Can you work these out from the model? Positions are in its coordinate system, mm. A direction names the side the tool comes from. Give positions to 0.01 mm unless a question says otherwise; leave off trailing zeros. Loops run counter-clockwise (first coordinate to the right, second up) from the corner with the lowest first, then second, coordinate; pieces in that order, holes last. Notation, with made-up numbers: (48.5, 60.5) -> (93.5, 60.5) arc R11 cw to (93.5, 66.5) -> close; hole circle Ø6 at (23, 1.25). An arc over 180 degrees is marked (long way). Use CSV: the item, a comma, the result in double quotes.
Autodesk Inventor part; units mm, degrees
ref_plane "YZ Plane" through (0, 0, 0) normal (1, 0, 0) x (0, 1, 0)
ref_plane "XZ Plane" through (0, 0, 0) normal (0, 1, 0) x (-1, 0, 0)
ref_plane "XY Plane" through (0, 0, 0) normal (0, 0, 1) x (1, 0, 0)
sketch "Sketch1" plane through (0, 0, 0) normal (0, 0, 1) x (1, 0, 0)
  line L0 (0, 53.34) -> (96.52, 53.34)
  line L1 (96.52, 53.34) -> (99.06, 50.8)
  line L2 (99.06, 50.8) -> (99.06, 40.64)
  line L3 (99.06, 40.64) -> (101.6, 38.1)
  line L4 (101.6, 38.1) -> (101.6, 3.81)
  line L5 (99.06, 0) -> (0, 0)
  line L6 (0, 0) -> (0, 53.34)
  line L7 (101.6, 3.81) -> (99.06, 1.27)
  line L8 (99.06, 1.27) -> (99.06, 0)
  line L9 (96.9093, 54.2798) -> (-0.9398, 54.2798)
  line L10 (-0.9398, 54.2798) -> (-0.9398, -0.9398)
  line L11 (-0.9398, -0.9398) -> (99.9998, -0.9398)
  line L12 (99.9998, -0.9398) -> (99.9998, 0.8807)
  line L13 (99.9998, 0.8807) -> (102.5398, 3.4207)
  line L14 (102.5398, 3.4207) -> (102.5398, 38.4893)
  line L15 (102.5398, 38.4893) -> (99.9998, 41.0293)
  line L16 (99.9998, 41.0293) -> (99.9998, 51.1893)
  line L17 (99.9998, 51.1893) -> (96.9093, 54.2798)
  line L18 (96.6042, 53.5432) -> (-0.2032, 53.5432)
  line L19 (-0.2032, 53.5432) -> (-0.2032, -0.2032)
  line L20 (-0.2032, -0.2032) -> (99.2632, -0.2032)
  line L21 (99.2632, -0.2032) -> (99.2632, 1.1858)
  line L22 (99.2632, 1.1858) -> (101.8032, 3.7258)
  line L23 (101.8032, 3.7258) -> (101.8032, 38.1842)
  line L24 (101.8032, 38.1842) -> (99.2632, 40.7242)
  line L25 (99.2632, 40.7242) -> (99.2632, 50.8842)
  line L26 (99.2632, 50.8842) -> (96.6042, 53.5432)
  point P0 (0, 0)
  dimension "d0" = 96.52
  dimension "d1" = 53.34
  dimension "d4" = 99.06
  dimension "d5" = 50.8
  dimension "d6" = 101.6
  dimension "d7" = 40.64
  dimension "d8" = 38.1
  dimension "d9" = 99.06
  dimension "d10" = 1.27
  dimension "d11" = 3.81
  dimension "d15" = 0.2032
  dimension "d18" = 0.7366
extrude "Extrusion2" add sketch "Sketch1" along normal blind 2.54 contours L17 L16 L15 L14 L13 L12 L11 L10 L9
sketch "Sketch2" plane through (0, 0, 0) normal (0, 0, 1) x (1, 0, 0)
  line L0 (0, 53.34) -> (96.52, 53.34)
  line L1 (96.52, 53.34) -> (99.06, 50.8)
  line L2 (99.06, 50.8) -> (99.06, 40.64)
  line L3 (99.06, 40.64) -> (101.6, 38.1)
  line L4 (101.6, 38.1) -> (101.6, 3.81)
  line L5 (99.06, 0) -> (0, 0)
  line L6 (0, 0) -> (0, 53.34)
  line L7 (101.6, 3.81) -> (99.06, 1.27)
  line L8 (99.06, 1.27) -> (99.06, 0)
  line L9 (96.9093, 54.2798) -> (-0.9398, 54.2798)
  line L10 (-0.9398, 54.2798) -> (-0.9398, -0.9398)
  line L11 (-0.9398, -0.9398) -> (99.9998, -0.9398)
  line L12 (99.9998, -0.9398) -> (99.9998, 0.8807)
  line L13 (99.9998, 0.8807) -> (102.5398, 3.4207)
  line L14 (102.5398, 3.4207) -> (102.5398, 38.4893)
  line L15 (102.5398, 38.4893) -> (99.9998, 41.0293)
  line L16 (99.9998, 41.0293) -> (99.9998, 51.1893)
  line L17 (99.9998, 51.1893) -> (96.9093, 54.2798)
  line L18 (96.6042, 53.5432) -> (-0.2032, 53.5432)
  line L19 (-0.2032, 53.5432) -> (-0.2032, -0.2032)
  line L20 (-0.2032, -0.2032) -> (99.2632, -0.2032)
  line L21 (99.2632, -0.2032) -> (99.2632, 1.1858)
  line L22 (99.2632, 1.1858) -> (101.8032, 3.7258)
  line L23 (101.8032, 3.7258) -> (101.8032, 38.1842)
  line L24 (101.8032, 38.1842) -> (99.2632, 40.7242)
  line L25 (99.2632, 40.7242) -> (99.2632, 50.8842)
  line L26 (99.2632, 50.8842) -> (96.6042, 53.5432)
  line L27 (4.1402, 4.1402) -> (4.1402, 49.1998)
  circle A0 centre (15.24, 50.8) radius 1.5875
  circle A1 centre (13.97, 2.54) radius 1.5875
  line L28 (13.7585, 47.9425) -> (16.8275, 47.9425)
  line L29 (16.8275, 47.9425) -> (18.0848, 49.1998)
  line L30 (13.7585, 47.9425) -> (12.5012, 49.1998)
  line L31 (4.1402, 49.1998) -> (12.5012, 49.1998)
  line L32 (18.0848, 49.1998) -> (87.3252, 49.1998)
  line L33 (12.3825, 5.3344) -> (15.5575, 5.3344)
  line L34 (15.5575, 5.3344) -> (16.7517, 4.1402)
  line L35 (12.3825, 5.3344) -> (11.1883, 4.1402)
  line L36 (91.8972, 4.1402) -> (16.7517, 4.1402)
  line L37 (11.1883, 4.1402) -> (4.1402, 4.1402)
  line L38 (91.8972, 46.2153) -> (91.8972, 4.1402)
  circle A2 centre (90.17, 50.8) radius 1.5875
  circle A3 centre (96.52, 2.54) radius 1.5875
  line L39 (90.17, 47.9425) -> (88.5825, 47.9425)
  line L40 (88.5825, 47.9425) -> (87.3252, 49.1998)
  line L41 (90.17, 47.9425) -> (91.8972, 46.2153)
  point P0 (0, 0)
  point P1 (0, 1.4137)
  dimension "d19" = 96.52
  dimension "d20" = 53.34
  dimension "d21" = 99.06
  dimension "d22" = 50.8
  dimension "d23" = 101.6
  dimension "d24" = 40.64
  dimension "d25" = 38.1
  dimension "d26" = 99.06
  dimension "d27" = 1.27
  dimension "d28" = 3.81
  dimension "d29" = 0.2032
  dimension "d30" = 0.7366
  dimension "d70" = 13.97
  dimension "d71" = 2.54
  dimension "d72" = 3.175
  dimension "d73" = 50.8
  dimension "d74" = 3.175
  dimension "d75" = 15.24
  dimension "d135" = 2.54
  dimension "d136" = 1.27
  dimension "d146" = 4.1402
  dimension "d148" = 91.8972
  dimension "d150" = 3.175
  dimension "d151" = 3.175
  dimension "d152" = 90.17
  dimension "d153" = 50.8
  dimension "d154" = 1.27
  dimension "d155" = 2.54
  dimension "d156" = 96.52
extrude "Extrusion3" add sketch "Sketch2" against normal blind 2.54 contours L0 L1 L2 L3 L4 L7 L8 L5 L6 | L17 L16 L15 L14 L13 L12 L11 L10 L9 | L26 L25 L24 L23 L22 L21 L20 L19 L18
sketch "Sketch4" plane through (0, 0, 2.54) normal (0, 0, 1) x (1, 0, 0)
  line L0 (-0.2032, -0.2032) -> (-0.2032, 53.5432)
  line L1 (-0.9398, -0.9398) -> (-0.9398, 54.2798)
  line L2 (-0.2032, 12.446) -> (-0.9398, 12.446)
  line L3 (-0.2032, 2.8575) -> (-0.9398, 2.8575)
  line L4 (-0.2032, 32.004) -> (-0.9398, 32.004)
  line L5 (-0.2032, 44.196) -> (-0.9398, 44.196)
  point P0 (0, 0)
  dimension "d35" = 12.446
  dimension "d36" = 2.8575
  dimension "d37" = 32.004
  dimension "d38" = 44.196
extrude "Extrusion4" cut sketch "Sketch4" against normal blind 2.286 contours L3 L1 L2 L0 | L4 L1 L5 L0
sketch "Sketch5" plane through (0, 0, 0) normal (0, 0, 1) x (1, 0, 0)
  line L0 (25.4, 3.3338) -> (92.71, 3.3338)
  line L1 (92.71, 3.3338) -> (92.71, 1.7463)
  line L2 (92.71, 1.7463) -> (25.4, 1.7463)
  line L3 (25.4, 1.7463) -> (25.4, 3.3338)
  line L4 (17.78, 51.5938) -> (87.63, 51.5938)
  line L5 (87.63, 51.5938) -> (87.63, 50.0063)
  line L6 (87.63, 50.0063) -> (17.78, 50.0062)
  line L7 (17.78, 50.0062) -> (17.78, 51.5938)
  line L8 (-0.2032, 53.5432) -> (-0.2032, -0.2032)
  line L9 (-0.2032, 12.065) -> (11.2268, 12.065)
  line L10 (11.2268, 12.065) -> (11.2268, 1.6002)
  line L11 (11.2268, 1.6002) -> (-0.2032, 1.6002)
  line L12 (-0.2032, 1.6002) -> (-0.2032, 12.065)
  line L13 (1.6002, 12.065) -> (1.6002, 1.6002)
  line L14 (4.1402, 4.1402) -> (4.1402, 49.1998)
  line L15 (4.1402, 49.1998) -> (12.5012, 49.1998)
  line L16 (91.8972, 4.1402) -> (16.7517, 4.1402)
  line L17 (99.2632, 50.8842) -> (96.6042, 53.5432)
  line L18 (96.6042, 53.5432) -> (-0.2032, 53.5432)
  line L19 (-0.2032, 53.5432) -> (-0.2032, -0.2032)
  line L20 (-0.2032, -0.2032) -> (99.2632, -0.2032)
  line L21 (99.2632, -0.2032) -> (99.2632, 1.1858)
  line L22 (99.2632, 1.1858) -> (101.8032, 3.7258)
  line L23 (101.8032, 3.7258) -> (101.8032, 38.1842)
  line L24 (101.8032, 38.1842) -> (99.2632, 40.7242)
  line L25 (99.2632, 40.7242) -> (99.2632, 50.8842)
  line L26 (91.8972, 4.1402) -> (16.7517, 4.1402)
  line L27 (4.1402, 4.1402) -> (4.1402, 49.1998)
  line L28 (1.6002, 44.4853) -> (4.1402, 47.0253)
  line L29 (99.2632, 40.7242) -> (99.2632, 50.8842)
  line L30 (1.6002, 31.7147) -> (4.1402, 29.1747)
  line L31 (1.6002, 31.7147) -> (1.6002, 44.4853)
  line L32 (4.1402, 47.0253) -> (4.1402, 29.1747)
  line L33 (12.5012, 49.1998) -> (13.7585, 47.9425)
  line L34 (13.7585, 47.9425) -> (16.8275, 47.9425)
  line L35 (16.8275, 47.9425) -> (18.0848, 49.1998)
  line L36 (18.0848, 49.1998) -> (87.3252, 49.1998)
  line L37 (11.1883, 4.1402) -> (4.1402, 4.1402)
  line L38 (16.7517, 4.1402) -> (15.5575, 5.3344)
  line L39 (15.5575, 5.3344) -> (12.3825, 5.3344)
  line L40 (12.3825, 5.3344) -> (11.1883, 4.1402)
  line L41 (15.5575, 5.3344) -> (12.3825, 5.3344)
  line L42 (97.79, 51.5938) -> (92.71, 51.5938)
  line L43 (92.71, 51.5938) -> (92.71, 6.35)
  line L44 (92.71, 6.35) -> (97.79, 6.35)
  line L45 (97.79, 6.35) -> (97.79, 51.5938)
  line L46 (91.8972, 46.2153) -> (91.8972, 4.1402)
  line L47 (87.3252, 49.1998) -> (88.5825, 47.9425)
  line L48 (88.5825, 47.9425) -> (90.17, 47.9425)
  line L49 (90.17, 47.9425) -> (91.8972, 46.2153)
  point P0 (0, 0)
  point P1 (61.8998, 4.1402)
  dimension "d41" = 1.5875
  dimension "d42" = 25.4
  dimension "d43" = 92.71
  dimension "d44" = 17.78
  dimension "d45" = 87.63
  dimension "d46" = 1.5875
  dimension "d47" = 51.5938
  dimension "d48" = 1.7463
  dimension "d51" = 0
  dimension "d52" = 12.065
  dimension "d54" = 11.43
  dimension "d97" = 2.54
  dimension "d101" = 2.54
  dimension "d102" = 2.54
  dimension "d142" = 5.08
  dimension "d143" = 0
  dimension "d145" = 6.35
  dimension "d149" = 92.71
extrude "Extrusion5" cut sketch "Sketch5" against normal blind 2.159 contours L0 L1 L2 L3 | L4 L5 L6 L7 | L45 L44 L43 L42
sketch "Sketch7" plane through (0, 0, 0) normal (0, 0, 1) x (1, 0, 0)
  line L0 (25.4, 3.3338) -> (64.77, 3.3338)
  line L1 (64.77, 3.3338) -> (64.77, 1.7463)
  line L2 (64.77, 1.7463) -> (25.4, 1.7463)
  line L3 (25.4, 1.7463) -> (25.4, 3.3338)
  line L4 (17.78, 51.5938) -> (64.77, 51.5938)
  line L5 (64.77, 51.5938) -> (64.77, 50.0062)
  line L6 (64.77, 50.0062) -> (17.78, 50.0062)
  line L7 (17.78, 50.0062) -> (17.78, 51.5938)
  line L8 (-0.2032, 53.5432) -> (-0.2032, -0.2032)
  line L9 (-0.2032, 12.065) -> (11.2268, 12.065)
  line L10 (11.2268, 12.065) -> (11.2268, 1.6002)
  line L11 (11.2268, 1.6002) -> (-0.2032, 1.6002)
  line L12 (-0.2032, 1.6002) -> (-0.2032, 12.065)
  line L13 (1.6002, 12.065) -> (1.6002, 1.6002)
  line L14 (63.627, 30.43) -> (66.167, 30.43) construction
  line L15 (63.627, 25.35) -> (63.627, 30.43) construction
  line L16 (66.167, 30.43) -> (66.167, 25.35) construction
  line L17 (66.167, 25.35) -> (63.627, 25.35) construction
  line L18 (4.1402, 4.1402) -> (4.1402, 49.1998)
  line L19 (4.1402, 49.1998) -> (61.8998, 49.1998)
  line L20 (61.8998, 49.1998) -> (61.8998, 38.6711)
  line L21 (61.8998, 38.6711) -> (64.4398, 36.1311)
  line L22 (64.4398, 6.866) -> (64.4398, 6.7949)
  line L23 (64.4398, 6.7949) -> (61.8998, 4.2549)
  line L24 (61.8998, 4.2549) -> (61.8998, 4.1402)
  line L25 (61.8998, 4.1402) -> (4.1402, 4.1402)
  line L26 (66.2432, 51.9002) -> (64.6002, 53.5432)
  line L27 (64.6002, 53.5432) -> (-0.2032, 53.5432)
  line L28 (-0.2032, 53.5432) -> (-0.2032, -0.2032)
  line L29 (-0.2032, -0.2032) -> (66.2432, -0.2032)
  line L30 (66.2432, -0.2032) -> (66.2432, 2.4558)
  line L31 (66.2432, 2.4558) -> (68.7832, 4.9958)
  line L32 (68.7832, 4.9958) -> (68.7832, 37.9302)
  line L33 (68.7832, 37.9302) -> (66.2432, 40.4702)
  line L34 (66.2432, 40.4702) -> (66.2432, 51.9002)
  line L35 (64.4398, 36.1311) -> (64.4398, 6.7949)
  line L36 (65.7098, 32.462) -> (66.9798, 31.192)
  line L37 (65.7098, 23.318) -> (66.9798, 24.588)
  line L38 (66.9798, 31.192) -> (66.9798, 24.588)
  line L39 (64.4398, 33.732) -> (64.4398, 22.048)
  line L40 (61.8998, 4.1402) -> (4.1402, 4.1402)
  line L41 (4.1402, 4.1402) -> (4.1402, 49.1998)
  line L42 (1.6002, 44.4853) -> (4.1402, 47.0253)
  line L43 (66.2432, 40.4702) -> (66.2432, 51.9002)
  line L44 (1.6002, 31.7147) -> (4.1402, 29.1747)
  line L45 (1.6002, 31.7147) -> (1.6002, 44.4853)
  line L46 (4.1402, 47.0253) -> (4.1402, 29.1747)
  arc A0 (64.4398, 8.374) -> (64.4398, 6.866) centre (65.8368, 7.62) ccw
  line L47 (64.4398, 36.1311) -> (64.4398, 8.374)
  line L48 (64.4398, 32.462) -> (65.7098, 32.462)
  line L49 (65.7098, 23.318) -> (65.0748, 23.318)
  line L50 (65.0748, 23.318) -> (64.4398, 22.683)
  point P0 (0, 0)
  point P1 (0, 0)
  point P2 (64.4398, 31.192)
  point P3 (64.4398, 31.192)
  point P4 (64.4398, 24.588)
  point P5 (64.4398, 24.588)
  dimension "d106" = 1.5875
  dimension "d107" = 25.4
  dimension "d108" = 64.77
  dimension "d109" = 17.78
  dimension "d110" = 64.77
  dimension "d111" = 1.5875
  dimension "d112" = 51.5938
  dimension "d113" = 1.7463
  dimension "d114" = 0
  dimension "d115" = 12.065
  dimension "d116" = 11.43
  dimension "d117" = 2.54
  dimension "d118" = 2.54
  dimension "d119" = 2.54
  dimension "d120" = 2.54
  dimension "d121" = 2.54
  dimension "d122" = 2.54
  dimension "d123" = 2.54
extrude "Extrusion7" cut sketch "Sketch7" against normal through all contours L9 L18 L25 L10 L11 L13 | L9 L10 L25 L18 | L44 L45 L42 L18 | L48 L36 L38 L37 L49 L50 L35
chamfer "Chamfer3" distance 2.54 angle 45 1 edges at (4.1402, 12.065, -1.27)
chamfer "Chamfer5" distance 2.54 angle 45 1 edges at (1.6002, 1.6002, -1.27)
chamfer "Chamfer6" distance 0.381 angle 45 8 edges at (12.3825, 2.54, 0) (13.6525, 50.8, 0) (13.6525, 50.8, -2.54) (12.3825, 2.54, -2.54) (94.9325, 2.54, -2.54) (88.5825, 50.8, -2.54) (88.5825, 50.8, 0) (94.9325, 2.54, 0)
equation "\"d97\" = d101"
equation "\"d102\" = d101"
properties part number "Arduino MEGA Bumper 0003"
(1) If I drill on L1, parallel to Y at x = 57, z = -1.4; L2, parallel to Y at x = 90.17, z = -1.25; L3, parallel to Y at x = 96.52, z = -1.5, over which ranges is the centre line in solid material (lowest first)? Write a range as from..to.
Answer sheet:
L1,"y = -0.94..1.75, 3.33..4.14, 49.2..50.01, 51.59..54.28"
L2,"y = -0.94..1.75, 3.33..4.14, 47.94..49.21, 52.39..54.28"
L3,"y = -0.94..0.95, 4.13..6.35, 51.59..54.28"
(2) Will these pins go through, and if not, where does the flat tip stop? pin 1 Ø3 at (x, y) = (90.17, 50.8) entering from -Z; pin 2 Ø0.8 at (x, y) = (65, 2.5) entering from +Z; pin 3 Ø2 at (y, z) = (41, -1.5) entering from +X.
Answer sheet:
pin 1,"passes through"
pin 2,"stops at z = -2.16"
pin 3,"stops at x = 101.03"
(3) If we section it at B-B, the plane x = 64.5: Write out the boundary of the cut face in (y, z), then the cut area to 3 significant figures.
Answer sheet:
outline,"(-0.94, -2.54) -> (4.14, -2.54) -> (4.14, 0) -> (3.33, 0) -> (3.33, -2.16) -> (1.75, -2.16) -> (1.75, 0) -> (-0.2, 0) -> (-0.2, 2.54) -> (-0.94, 2.54) -> close; (49.2, -2.54) -> (54.28, -2.54) -> (54.28, 2.54) -> (53.54, 2.54) -> (53.54, 0) -> (51.59, 0) -> (51.59, -2.16) -> (50.01, -2.16) -> (50.01, 0) -> (49.2, 0) -> close"
area,"22.7 mm2"
(4) We'd pull the mould along Y, two halves only. Please class faces 4 (the face through (101.29, 39.74, -0.04)), 5 (the face through (88.584, 50.87, -1.258)), 6 (the face through (100, 0, 0)): released by +Y, released by -Y, zero draft, split by the parting line, or undercut.
Answer sheet:
face 4,"released by +Y"
face 5,"undercut"
face 6,"zero draft"
(5) Which directions (+Z, -Z, +X, -X, +Y, -Y) give clear straight access to the entire face, cutting with the end or side of a thin tool? Please do faces 1 (the face through (49, 54.28, 0)), 2 (the face through (1.6, 8, -1)), 3 (the face through (92.71, 29, -1)).
Answer sheet:
face 1,"+Z, -Z, +X, -X, +Y"
face 2,"+Z, -Z"
face 3,"+Z"
(6) If we section it at C-C, the plane y = 27.5: Write out the boundary of the cut face in (x, z).
Answer sheet:
outline,"(-0.94, -2.54) -> (4.14, -2.54) -> (4.14, 0) -> (-0.2, 0) -> (-0.2, 2.54) -> (-0.94, 2.54) -> close; (91.9, -2.54) -> (102.54, -2.54) -> (102.54, 2.54) -> (101.8, 2.54) -> (101.8, 0) -> (97.79, 0) -> (97.79, -2.16) -> (92.71, -2.16) -> (92.71, 0) -> (91.9, 0) -> close"
(7) If we section it at A-A, the plane y = 34: Write out the boundary of the cut face in (x, z).
Answer sheet:
outline,"(-0.94, -2.54) -> (1.6, -2.54) -> (1.6, 0) -> (-0.2, 0) -> (-0.2, 0.25) -> (-0.94, 0.25) -> close; (91.9, -2.54) -> (102.54, -2.54) -> (102.54, 2.54) -> (101.8, 2.54) -> (101.8, 0) -> (97.79, 0) -> (97.79, -2.16) -> (92.71, -2.16) -> (92.71, 0) -> (91.9, 0) -> close"
